Check sheet for the modelled part. Datum: model origin and axes. Units: mm. Face numbers are marked on the shaded views. A direction names the side the tool comes from. Coordinates: 2 decimals unless noted, no trailing zeros. Order: outer loops, then holes, each group sorted by start corner. A loop starts at its lowest first (then second) coordinate and runs counter-clockwise, first axis right, second up.
1. Cross-section at B-B (x = -35.5). Enter the section's corners in (y, z), then the cut area to 3 significant figures.
2. Cross-section at C-C (z = 31.5). Enter the section's corners in (x, y).
3. Gauge pin test, flat ends, axial feed: pin 1 Ø10 at (y, z) = (22, 29) entering from -X; pin 2 Ø12 at (x, y) = (-1, 26.5) entering from +Z; pin 3 Ø2 at (x, z) = (41.5, -6.5) entering from +Y; pin 4 Ø1.5 at (x, y) = (9, 4) entering from -Z. Record the tip position at first contact, or that the pin passes through.
4. Draft check along Z on the marked faces 1, 2 and 3. Enter one of: released by +Z, released by -Z, zero draft, split by the parting line, or undercut.
5. Cross-section at D-D (y = 22.5). Enter the section's corners in (x, z), then the cut area to 4 significant figures.
6. Cross-section at A-A (y = -5). Count the separate pieces of the cut face and the enclosed holes in it, then the cut area to 3 significant figures.
7. Set-up check for the marked faces 4, 5, 6 and 7: record each of +Z, -Z, +X, -X, +Y, -Y from which the full face is reachable in a straight line by a thin tool's end or side.
8. Thickness scan on line 1 (Z direction, x = -51, y = -7); line 2 (Y direction, x = 54, z = 7.5); line 3 (Y direction, x = -35, z = 32.5). Record the ranges inside material, lowest first.
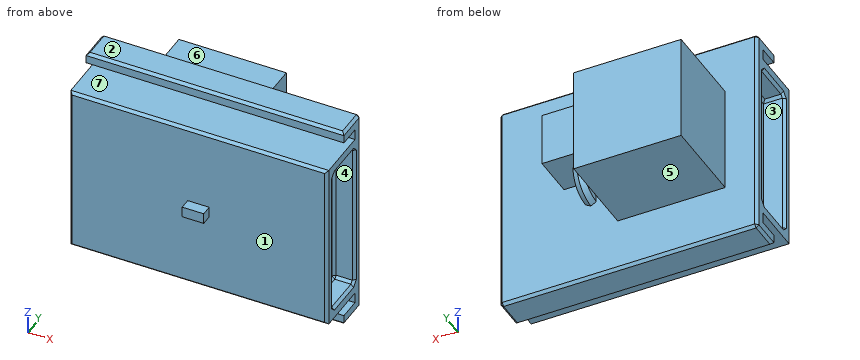
```python
from build123d import *

# Parameters (mm, degrees)
BOSS_EXTRUDE1_DEPTH = 60
SKETCH2_W           = 50
SKETCH2_H           = 50
BOSS_EXTRUDE2_DEPTH = 40
SKETCH2_3_W         = 25
SKETCH2_3_H         = 25
BOSS_EXTRUDE3_DEPTH = 20
SKETCH7_W           = 70
SKETCH7_H           = 20
CUT_EXTRUDE1_DEPTH  = 10
SKETCH8_W           = 10
SKETCH8_H           = 5
BOSS_EXTRUDE4_DEPTH = 5
CHAMFER1_SIZE       = 1.25


with BuildPart() as part:
    # Sketch1 → Boss-Extrude1 (new body, symmetric)
    with BuildSketch(Plane(origin=(0, 0, 0), x_dir=(0, 0, -1), z_dir=(1, 0, 0))):
        Polygon((-40, 0), (-45, 0), (-45, -10), (-50, -10), (-50, 5), (50, 5), (50, -10), (45, -10), (45, 0), (40, 0), (40, -25), (-40, -25), align=None)
    extrude(amount=BOSS_EXTRUDE1_DEPTH, both=True)

    # Sketch2 → Boss-Extrude2 (add)
    with BuildSketch(Plane(origin=(0, 5, 0), x_dir=(1, 0, 0), z_dir=(0, 1, 0))):
        with Locations((-20, 0)):
            Rectangle(SKETCH2_W, SKETCH2_H)
    extrude(amount=BOSS_EXTRUDE2_DEPTH)

    # Sketch2<3> → Boss-Extrude3 (add)
    with BuildSketch(Plane(origin=(0, 5, 0), x_dir=(1, 0, 0), z_dir=(0, 1, 0))):
        with Locations((17.5, -12.5)):
            Rectangle(SKETCH2_3_W, SKETCH2_3_H)
    extrude(amount=BOSS_EXTRUDE3_DEPTH)

    # Sketch3 → Loft3 section 0
    with BuildSketch(Plane(origin=(0, 0, 0), x_dir=(-1, 0, 0), z_dir=(0, 0, -1))):
        Polygon((-17.5, 17.886751346), (-20, 16.443375673), (-20, 13.556624327), (-17.5, 12.113248654), (-15, 13.556624327), (-15, 16.443375673), align=None)
    # Sketch6 → Loft3 section 1
    with BuildSketch(Plane(origin=(0, 2.5, 2.5), x_dir=(1, 0, 0), z_dir=(0, 0.707106781, 0.707106781))):
        Polygon((17.5, 16.422285252), (15, 14.978909579), (15, 12.092158233), (17.5, 10.64878256), (20, 12.092158233), (20, 14.978909579), align=None)
    # Sketch4 → Loft3 section 2
    with BuildSketch(Plane(origin=(0, 5, 0), x_dir=(1, 0, 0), z_dir=(0, 1, 0))):
        Polygon((17.5, 12.886751346), (15, 11.443375673), (15, 8.556624327), (17.5, 7.113248654), (20, 8.556624327), (20, 11.443375673), align=None)
    loft()

    # Sketch7 → Cut-Extrude1 (cut)
    with BuildSketch(Plane(origin=(60, 0, 0), x_dir=(0, 0, -1), z_dir=(1, 0, 0))):
        with Locations((0, -10)):
            Rectangle(SKETCH7_W, SKETCH7_H)
    cut_extrude1 = extrude(amount=-CUT_EXTRUDE1_DEPTH, mode=Mode.SUBTRACT)

    # Mirror1: Cut-Extrude1 across plane
    add(cut_extrude1.mirror(Plane(origin=(0, 0, 0), x_dir=(0, 0, 1), z_dir=(1, 0, 0))), mode=Mode.SUBTRACT)

    # Sketch8 → Boss-Extrude4 (add)
    with BuildSketch(Plane.XZ.offset(25)):
        Rectangle(SKETCH8_W, SKETCH8_H)
    extrude(amount=BOSS_EXTRUDE4_DEPTH)

    # Chamfer1
    chamfer1_edges = [part.edges().sort_by_distance(p)[0] for p in [
        (50, 0, 0),
        (55, 0, 35),
        (50, -10, -35),
        (55, 0, -35),
        (50, -20, 0),
        (55, -20, -35),
        (50, -10, 35),
        (55, -20, 35),
        (60, 0, 0),
        (60, -10, 35),
        (60, -20, 0),
        (60, -10, -35),
        (-60, 0, 0),
        (-55, 0, -35),
        (-60, -2.5, 50),
        (-60, -10, 35),
        (-55, 0, 35),
        (-60, -20, 0),
        (-55, -20, 35),
        (-60, -10, -35),
        (-55, -20, -35),
        (-50, -10, 35),
        (-50, -10, -35),
        (-60, 5, 0),
        (-60, -2.5, -50),
        (-60, -25, 0),
        (0, -10, 50),
        (0, 5, 50),
        (0, 5, -50),
        (0, -10, -50),
        (0, -25, -40),
        (0, -25, 40),
        (60, -2.5, -50),
        (60, 5, 0),
        (60, -2.5, 50),
        (60, -25, 0),
    ]]
    chamfer(chamfer1_edges, length=CHAMFER1_SIZE)


solid = part.part
```
Data:
1. outline: (-25, -38.75) - (-23.75, -40) - (0, -40) - (0, -45) - (-10, -45) - (-10, -48.75) - (-8.75, -50) - (3.75, -50) - (5, -48.75) - (5, -25) - (45, -25) - (45, 25) - (5, 25) - (5, 48.75) - (3.75, 50) - (-8.75, 50) - (-10, 48.75) - (-10, 45) - (0, 45) - (0, 40) - (-23.75, 40) - (-25, 38.75) - close
1. area: 4,600 mm2
2. outline: (-60, -23.75) - (-58.75, -25) - (58.75, -25) - (60, -23.75) - (60, -21.25) - (58.75, -20) - (51.25, -20) - (50, -18.75) - (50, -1.25) - (51.25, 0) - (58.75, 0) - (60, 1.25) - (60, 3.75) - (58.75, 5) - (-58.75, 5) - (-60, 3.75) - (-60, 1.25) - (-58.75, 0) - (-50, 0) - (-50, -20) - (-58.75, -20) - (-60, -21.25) - close
3. pin 1: stops at x = -45
3. pin 2: stops at z = 25
3. pin 3: stops at y = 5
3. pin 4: stops at z = -50
4. face 1: zero draft
4. face 2: released by +Z
4. face 3: undercut
5. outline: (-45, -25) - (5, -25) - (5, 0) - (30, 0) - (30, 25) - (-45, 25) - close
5. area: 3,125 mm2
6. separate pieces: 3
6. enclosed holes: 0
6. area: 9,400 mm2
7. face 4: +X
7. face 5: -Z, +X, -X, +Y
7. face 6: +Z, +X, -X, +Y
7. face 7: +X, -X, -Y
8. line 1: z = -50 to -45, -40 to -34.75, 34.75 to 40, 45 to 50
8. line 2: y = -25 to -20, 0 to 5
8. line 3: y = -25 to 5
